Read the model definition and answer for the solid it produces. Units are mm, in the model's axes. A direction names the side the tool comes from. Coordinates: 2 decimals unless noted, no trailing zeros. Order: outer loops, then holes, each group sorted by start corner. A loop starts at its lowest first (then second) coordinate and runs counter-clockwise, first axis right, second up. Notation, with made-up numbers: M 31,-2 L 44,-2 A17 ccw 44,16 Z; hole C 39,-34 d3. An arc over 180 degrees is marked long. Write each question's results on one line, items separated by ' | '.
```python
from build123d import *

# Parameters (mm, degrees)
F0_R     = 19.05
F1_DEPTH = 114.3
F2_R     = 10.16
F3_DEPTH = 25.4
F4_R     = 10.16
F5_DEPTH = 25.4


with BuildPart() as f1:
    # F0 (on Front) → F1 (new body, symmetric)
    with BuildSketch(Plane.XZ):
        Circle(F0_R)
    extrude(amount=F1_DEPTH, both=True)

    # F2 (on face) → F3 (join)
    with BuildSketch(Plane(origin=(0, 114.3, 0), x_dir=(-1, 0, 0), z_dir=(0, 1, 0))):
        Circle(F2_R)
    extrude(amount=F3_DEPTH)

    # F4 (on face) → F5 (join)
    with BuildSketch(Plane.XZ.offset(114.3)):
        Circle(F4_R)
    extrude(amount=F5_DEPTH)


solid = f1.part
```
(1) The part is cut by section A-A, the plane z = 0. Write down the section's boundary in (x, y), then the cut area to 3 significant figures.
Conclusion:
outline: M -19.05,-114.3 L -10.16,-114.3 L -10.16,-139.7 L 10.16,-139.7 L 10.16,-114.3 L 19.05,-114.3 L 19.05,114.3 L 10.16,114.3 L 10.16,139.7 L -10.16,139.7 L -10.16,114.3 L -19.05,114.3 Z | area: 9,740 mm²
(2) The part is cut by section B-B, the plane x = 0. Write down the section's boundary in (y, z).
Conclusion:
outline: M -139.7,-10.16 L -114.3,-10.16 L -114.3,-19.05 L 114.3,-19.05 L 114.3,-10.16 L 139.7,-10.16 L 139.7,10.16 L 114.3,10.16 L 114.3,19.05 L -114.3,19.05 L -114.3,10.16 L -139.7,10.16 Z
(3) Straight lines are drawn through the part: line 1 (Y direction, x = 10.5, z = 0.5); line 2 (Z direction, x = 0.5, y = 93); line 3 (X direction, y = -10.5, z = -6). For each, find the intervals that lie inside material, in ascending order.
Conclusion:
line 1: -114.3 to 114.3 | line 2: -19.04 to 19.04 | line 3: -18.08 to 18.08
(4) The part is cut by section D-D, the plane z = 16.5. Write down the section's boundary in (x, y), then the cut area to 3 significant figures.
Conclusion:
outline: M -9.52,-114.3 L 9.52,-114.3 L 9.52,114.3 L -9.52,114.3 Z | area: 4,350 mm²
(5) For faces 1 (the cylindrical face through (-1.323, -126.822, 10.074)), 2 (the flat face through (0, -139.7, 0)), 3 (the flat face through (8, 114.3, -8)), determine the directions among +Z, -Z, +X, -X, +Y, -Y from which every point of the face is accessible in a straight line to the end or side of a thin tool.
Conclusion:
face 1: -Y | face 2: +Z, -Z, +X, -X, -Y | face 3: +Y
(6) The part is cut by section C-C, the plane y = -40. Write down the section's boundary in (x, z).
Conclusion:
outline: C 0,0 d38.1
(7) Given pin 1 (1 mm diameter, centred on y = 99, z = 6.5, fed in from -X); pin 2 (2 mm diameter, centred on x = -12.5, z = 0, fed in from -Y); pin 3 (5 mm diameter, centred on x = -4.5, y = 31.5, fed in from +Z), each flat-ended and moving along its own axis, determine where each tip first touches the part or whether it passes through.
Conclusion:
pin 1: x = -18.08 | pin 2: y = -114.3 | pin 3: z = 18.94
